Model file for the job. Use its own axes, mm. A direction names the side the tool comes from. Coordinates: 2 decimals unless noted, no trailing zeros. Write each loop counter-clockwise with the first axis right and the second up, starting at its lowest first coordinate (ties: lowest second). Pieces come first, ordered by that corner, then holes. Notation, with made-up numbers: (53, -2.5) -> (58, -2.5) arc R22 ccw to (58, 15.5) -> close; hole circle Ø2 at (64, -21.75). An arc over 180 degrees is marked (long way). Answer as a JSON object with one key per item and string values. Group by question number.
Autodesk Inventor part; units mm, degrees
ref_plane "YZ Plane" through (0, 0, 0) normal (1, 0, 0) x (0, 1, 0)
ref_plane "XZ Plane" through (0, 0, 0) normal (0, 1, 0) x (-1, 0, 0)
ref_plane "XY Plane" through (0, 0, 0) normal (0, 0, 1) x (1, 0, 0)
sketch "Sketch1" plane through (0, 0, 0) normal (0, 0, 1) x (1, 0, 0)
  circle A0 centre (0, 0) radius 4
  circle A1 centre (0, 0) radius 3.9492
  circle A2 centre (0, 0) radius 5.2192
  circle A3 centre (0, 0) radius 3.175
  point P0 (0, 0)
  dimension "d0" = 0.0508
  dimension "d1" = 1.27
  dimension "d2" = 6.35
extrude "Extrusion1" add sketch "Sketch1" along normal blind 1.27 contours A0 | A1 | A2
extrude "Extrusion2" add sketch "Sketch1" against normal blind 8.5875 contours A1
chamfer "Chamfer1" distance 0.635 angle 45 1 edges at (-3.175, 0, 1.27)
properties part number "AxleAdapter"
(1) Cut at C-C on z = -6.75. List the corners of the cut face in (x, y) (3 decimals).
(2) Pull direction X, two halves, no side cores. Call faces 3 (the face through (-0.69, 3.1, -4.04)), 4 (the face through (1.822, -3.504, -4.234)), 5 (the face through (0, -4, 1.27)): released by +X, released by -X, zero draft, split by the parting line, or undercut.
(3) Cut at A-A on y = 0. List the corners of the cut face in (x, z) (1 decimal).
(4) 3-axis set-ups, long thin cutter, end or side, ignore diameter. For faces 1 (the face through (-1, 4, 0)), 2 (the face through (-3, 2, -8.588)): which of +Z, -Z, +X, -X, +Y, -Y reach the whole face in a straight line?
(5) Pin check, flat tips, straight feed: pin 1 (4 mm diameter, centred on x = 3, z = -7, fed in from -Y); pin 2 (1.5 mm diameter, centred on y = 2.5, z = -1, fed in from +X); pin 3 (2 mm diameter, centred on x = -0.5, z = -3, fed in from +Y). Stop position of each tip, or through.
(6) Wall check: probe 1 along Y at (x, z) = (0, -2.25) (3 decimals); probe 2 along Z at (x, y) = (-4, 1); probe 3 along Y at (x, z) = (0.75, -3.5). Give the ranges that are in metal, low to high.
Results found:
{
 "1": {"outline": "circle Ø7.898 at (0, 0); hole circle Ø6.35 at (0, 0)"},
 "2": {"face 3": "undercut", "face 4": "split by the parting line", "face 5": "zero draft"},
 "3": {"outline": "(-5.2, 0) -> (-3.9, 0) -> (-3.9, -8.6) -> (-3.2, -8.6) -> (-3.2, 0.6) -> (-3.8, 1.3) -> (-5.2, 1.3) -> close; (3.2, -8.6) -> (3.9, -8.6) -> (3.9, 0) -> (5.2, 0) -> (5.2, 1.3) -> (3.8, 1.3) -> (3.2, 0.6) -> close"},
 "4": {"face 1": "-Z", "face 2": "-Z, +X, -X, +Y, -Y"},
 "5": {"pin 1": "stops at y = -3.82", "pin 2": "stops at x = 3.54", "pin 3": "stops at y = 3.95"},
 "6": {"probe 1": "y = -3.949 to -3.175, 3.175 to 3.949", "probe 2": "z = 0 to 1.27", "probe 3": "y = -3.88 to -3.09, 3.09 to 3.88"}
}
